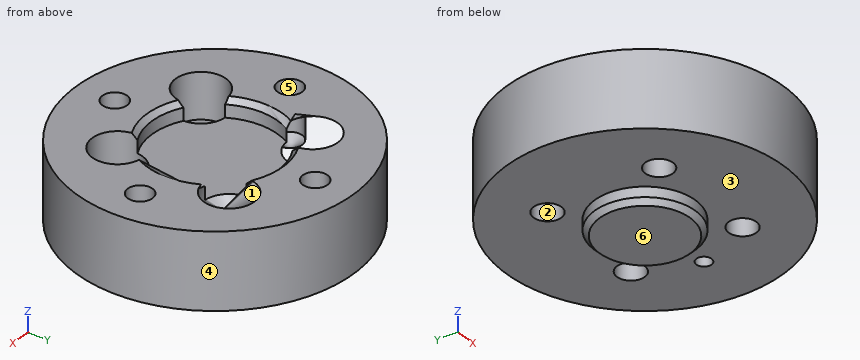
Autodesk Inventor part; units mm, degrees
ref_plane "YZ Plane" through (0, 0, 0) normal (1, 0, 0) x (0, 1, 0)
ref_plane "XZ Plane" through (0, 0, 0) normal (0, 1, 0) x (-1, 0, 0)
ref_plane "XY Plane" through (0, 0, 0) normal (0, 0, 1) x (1, 0, 0)
sketch "Sketch1" plane through (0, 0, 0) normal (0, 0, 1) x (1, 0, 0)
  circle A0 centre (0, 0) radius 27.5
  dimension "d0" = 55
extrude "Extrusion1" add sketch "Sketch1" along normal blind 15
sketch "Sketch2" plane through (0, 0, 15) normal (0, 0, 1) x (1, 0, 0)
  circle A0 centre (0, 0) radius 27.5
  circle A1 centre (0, 0) radius 12.5
  point P0 (15.75, 0)
  point P1 (20, 0)
  point P2 (11.1369, 11.1369)
  point P3 (0, 15.75)
  point P4 (-11.1369, 11.1369)
  point P5 (-15.75, 0)
  point P6 (-11.1369, -11.1369)
  point P7 (0, -15.75)
  point P8 (11.1369, -11.1369)
  point P9 (14.1421, 14.1421)
  point P10 (0, 20)
  point P11 (-14.1421, 14.1421)
  point P12 (-20, 0)
  point P13 (-14.1421, -14.1421)
  point P14 (0, -20)
  point P15 (14.1421, -14.1421)
  dimension "d3" = 15.75
  dimension "d4" = 20
  dimension "d7" = 360
  dimension "d11" = 360
  dimension "d13" = 25
extrude "Extrusion2" cut sketch "Sketch2" against normal blind 3.5 contours A1
hole "Hole1" at (-11.1369, 11.1369, 15) at (-11.1369, -11.1369, 15) at (11.1369, 11.1369, 15) at (11.1369, -11.1369, 15) direction (0, 0, -1) diameter 5.5 end through all counterbore diameter 10 counterbore depth 9
hole "Hole2" at (0, 20, 15) at (-20, 0, 15) at (0, -20, 15) at (20, 0, 15) direction (0, 0, -1) diameter 4.917 depth 10 tip angle 118
sketch "Sketch3" plane through (0, 0, 0) normal (0, 0, -1) x (-1, 0, 0)
  circle A0 centre (0, 0) radius 27.5
  circle A1 centre (0, 0) radius 10
  point P0 (-15.75, 0)
  dimension "d31" = 15.75
  dimension "d32" = 20
hole "Hole3" at (15.75, 0, 0) direction (0, 0, 1) diameter 3 depth 4 tip angle 118
extrude "Extrusion3" add sketch "Sketch3" along normal blind 3 contours A1
chamfer "Chamfer1" distance 1 angle 45 1 edges at (10, 0, -3)
chamfer "Chamfer2" distance 1 angle 45 4 edges at (12.5, 0, 15) (0, 12.5, 15) (0, -12.5, 15) (-12.5, 0, 15)
properties part number "plate_cfs055ca501u"
Verification items for the finished model (mm, model axes). Face numbers are marked on the shaded views. A direction names the side the tool comes from. Round coordinates to 2 decimals unless told otherwise and drop trailing zeros. Write each loop counter-clockwise with the first axis right and the second up, starting at its lowest first coordinate (ties: lowest second). Pieces come first, ordered by that corner, then holes. Notation, with made-up numbers: (35.5, 39) -> (64.5, 39) arc R11 ccw to (64.5, 48) -> close; hole circle Ø5 at (-27.5, 45.5). An arc over 180 degrees is marked (long way). Write each question's results on one line, items separated by ' | '. Start each with the question number.
1. Cross-section at A-A (z = 7.5). Count the separate pieces of the cut face and the enclosed holes in it, then the cut area to 3 significant figures.
2. Set-up check for the marked faces 1, 2 and 3: record each of +Z, -Z, +X, -X, +Y, -Y from which the full face is reachable in a straight line by a thin tool's end or side.
3. Material ranges on probe 1 along X at (y, z) = (7, 10); probe 2 along Y at (x, z) = (9, 3.75); probe 3 along Y at (x, z) = (-9, 6.5), recorded low to high. Write a range as from..to.
4. Draft check along X on the marked faces 4, 5 and 6. Enter one of: +X half, -X half, draft (parallel to the pull), parting line (faces both ways), or undercut.
5. Depth check by flat-ended pin: P1, Ø4.5, axis at x = -20, y = 0, coming from the +Z side; P2, Ø10, axis at x = -15.5, z = 14, coming from the +Y side; P3, Ø3, axis at x = -13, z = 14, coming from the -Y side. Enter the tip coordinate at first touch or a pass-through.
6. Cross-section at B-B (x = 23.5). Enter the section's corners in (y, z), then the cut area to 3 significant figures.
Solutions:
1) separate pieces: 1 | enclosed holes: 8 | area: 1,990 mm2
2) face 1: +Z | face 2: +Z, -Z | face 3: -Z
3) probe 1: x = -26.59..-13.95, -8.33..8.33, 13.95..26.59 | probe 2: y = -25.99..-12.87, -9.41..9.41, 12.87..25.99 | probe 3: y = -25.99..-15.66, -6.62..6.62, 15.66..25.99
4) face 4: parting line | face 5: undercut | face 6: draft
5) P1: stops at z = 4.87 | P2: stops at y = 25.42 | P3: stops at y = -24.98
6) outline: (-14.28, 0) -> (14.28, 0) -> (14.28, 15) -> (-14.28, 15) -> close | area: 428 mm2
